Could you check a few things on this model? Use its own coordinates, in mm. A direction names the side the tool comes from. Round coordinates to 2 decimals unless told otherwise and drop trailing zeros. Write each loop counter-clockwise with the first axis right and the second up, starting at its lowest first coordinate (ties: lowest second). Pieces come first, ordered by that corner, then holes. Notation, with made-up numbers: (83, -12.75) -> (111, -12.75) arc R14 cw to (111, 12.25) -> close; hole circle Ø7 at (31, 30.5). An arc over 180 degrees is marked (long way). Return JSON: item names as keys, results as strings.
from build123d import *

# Parameters (mm, degrees)
F0_W      = 234.95
F0_H      = 76.2
F1_DEPTH  = 12.7
F2_W      = 6.35
F2_H      = 6.35
F3_DEPTH  = 234.951
F5_DEPTH  = 76.201
F6_W      = 6.35
F6_H      = 63.5
F7_DEPTH  = 6.35
F8_W      = 6.35
F8_H      = 6.35
F9_DEPTH  = 166.135738
F10_W     = 6.35
F10_H     = 6.35
F11_DEPTH = 166.135738


with BuildPart() as f1:
    # F0 (on Right) → F1 (new body)
    with BuildSketch(Plane.YZ):
        with Locations((0, 38.1)):
            Rectangle(F0_W, F0_H)
    extrude(amount=F1_DEPTH)

    # F2 (on face) → F3 (cut, through all)
    with BuildSketch(Plane(origin=(0, 117.475, 0), x_dir=(-1, 0, 0), z_dir=(0, 1, 0))):
        with Locations((-3.175, 9.525)):
            Rectangle(F2_W, F2_H)
    extrude(amount=-F3_DEPTH, mode=Mode.SUBTRACT)

    # F4 (on face) → F5 (cut, through all)
    with BuildSketch(Plane.XY.offset(76.2)):
        Polygon((0, 104.775), (12.7, 117.475), (0, 117.475), align=None)
        Polygon((0, -104.775), (0, -117.475), (12.7, -117.475), align=None)
    extrude(amount=-F5_DEPTH, mode=Mode.SUBTRACT)

    # F6 (on face) → F7 (cut)
    with BuildSketch(Plane(origin=(0, 0, 0), x_dir=(0, -1, 0), z_dir=(-1, 0, 0))):
        with Locations((0, 44.45)):
            Rectangle(F6_W, F6_H)
    extrude(amount=-F7_DEPTH, mode=Mode.SUBTRACT)

    # F8 (on face) → F9 (cut, through all)
    with BuildSketch(Plane(origin=(-52.3875, -52.3875, 0), x_dir=(0.707107, -0.707107, 0), z_dir=(-0.707107, -0.707107, 0))):
        with Locations((88.872625, 53.975)):
            Rectangle(F8_W, F8_H)
        with Locations((88.872625, 22.225)):
            Rectangle(F8_W, F8_H)
    extrude(amount=-F9_DEPTH, mode=Mode.SUBTRACT)

    # F10 (on face) → F11 (cut, through all)
    with BuildSketch(Plane(origin=(-52.3875, 52.3875, 0), x_dir=(-0.707107, -0.707107, 0), z_dir=(-0.707107, 0.707107, 0))):
        with Locations((-88.872625, 53.975)):
            Rectangle(F10_W, F10_H)
        with Locations((-88.872625, 22.225)):
            Rectangle(F10_W, F10_H)
    extrude(amount=-F11_DEPTH, mode=Mode.SUBTRACT)


solid = f1.part
1) I want a section at B-B, the plane y = -80.5. Please give me the cut outline in (x, z).
Return value:
{"outline": "(0, 0) -> (12.7, 0) -> (12.7, 76.2) -> (0, 76.2) -> (0, 12.7) -> (6.35, 12.7) -> (6.35, 6.35) -> (0, 6.35) -> close"}
2) For faces 1 (the face through (10.424, 110.771, 53.931)), 2 (the face through (10.424, -110.771, 53.931)), 3 (the face through (3, -3.175, 44)), 4 (the face through (0, 53, 45)), 5 (the face through (3, -56, 12.7)), which set-ups out of +Z, -Z, +X, -X, +Y, -Y let a thin tool reach every point of the face, with its end or its side?
Return value:
{"face 1": "+X, +Y", "face 2": "+X, -Y", "face 3": "+Z, -X", "face 4": "+Z, -Z, -X, +Y, -Y", "face 5": "-X, +Y, -Y"}
3) I want a section at C-C, the plane z = 60. Please give me the cut outline in (x, y) (3 decimals), and give its area (3 significant figures).
Return value:
{"outline": "(0, -104.775) -> (12.7, -117.475) -> (12.7, 117.475) -> (0, 104.775) -> (0, 3.175) -> (6.35, 3.175) -> (6.35, -3.175) -> (0, -3.175) -> close", "area": "2,780 mm²"}
4) If I drill on probe 1 along Z at (x, y) = (5.75, -101.5); probe 2 along Y at (x, z) = (2, 61) (3 decimals), over which ranges is the centre line in solid material (lowest first)? Write a range as [from, to].
Return value:
{"probe 1": "[0, 6.35], [12.7, 76.2]", "probe 2": "[-106.775, -3.175], [3.175, 106.775]"}
5) Will these pins go through, and if not, where does the flat tip stop? pin 1 Ø3 at (x, z) = (9, 43.5) entering from +Y (3 decimals); pin 2 Ø7 at (x, z) = (4.5, 58.5) entering from -Y (3 decimals); pin 3 Ø1.9 at (x, z) = (4, 60) entering from +Y (3 decimals).
Return value:
{"pin 1": "y = 115.275", "pin 2": "y = -112.775", "pin 3": "y = 109.725"}
6) Thinking about a two-plate mould opening in Z: for faces 6 (the face through (11, 114, 25.4)), 7 (the face through (8, -2, 76.2)), 8 (the face through (0, -55, 45)), 9 (the face through (11, 114, 50.8)), which applies, pulls with the +Z half, pulls with the -Z half, needs draft (parallel to the pull), parting line crosses it, or undercut?
Return value:
{"face 6": "undercut", "face 7": "pulls with the +Z half", "face 8": "needs draft", "face 9": "undercut"}
7) I want a section at A-A, the plane x = 3. Please give me the cut outline in (y, z) (3 decimals).
Return value:
{"outline": "(-107.775, 0) -> (107.775, 0) -> (107.775, 6.35) -> (-107.775, 6.35) -> close; (-107.775, 12.7) -> (-3.175, 12.7) -> (-3.175, 76.2) -> (-107.775, 76.2) -> close; (3.175, 12.7) -> (107.775, 12.7) -> (107.775, 76.2) -> (3.175, 76.2) -> close"}
